CAD build for the part. Positions are in the model's coordinates, mm. A direction names the side the tool comes from. Coordinates: 2 decimals unless noted, no trailing zeros. Order: outer loops, then holes, each group sorted by start corner. A loop starts at its lowest first (then second) coordinate and runs counter-clockwise, first axis right, second up. Notation, with made-up numbers: M 42.25,-20 L 95.25,-20 A21 cw 95.25,3 Z; hole C -3.75,7 d6. An arc over 180 degrees is marked long. Write item = value, one per line. Start each with the question number.
```python
from build123d import *

# Parameters (mm, degrees)
SKETCH_R        = 17.5
PAD_DEPTH       = 58
FILLET_R        = 15
SKETCH001_R     = 14.25
POCKET_DEPTH    = 32
SKETCH002_R     = 1
POCKET001_DEPTH = 58.001
FILLET001_R     = 2


with BuildPart() as part:
    # Sketch → Pad (new body)
    with BuildSketch(Plane.XY):
        Circle(SKETCH_R)
    extrude(amount=PAD_DEPTH)

    # Fillet
    fillet_edges = [part.edges().sort_by_distance(p)[0] for p in [
        (-17.5, 0, 58),
    ]]
    fillet(fillet_edges, radius=FILLET_R)

    # Sketch001 (on Face3 of Fillet) → Pocket (cut)
    with BuildSketch(Plane(origin=(0, 0, 0), x_dir=(1, 0, 0), z_dir=(0, 0, -1))):
        Circle(SKETCH001_R)
    extrude(amount=-POCKET_DEPTH, mode=Mode.SUBTRACT)

    # Sketch002 (on Face4 of Fillet) → Pocket001 (cut, through all)
    with BuildSketch(Plane.XY.offset(58)):
        Circle(SKETCH002_R)
    extrude(amount=-POCKET001_DEPTH, mode=Mode.SUBTRACT)

    # Fillet001
    fillet001_edges = [part.edges().sort_by_distance(p)[0] for p in [
        (-14.25, 0, 0),
    ]]
    fillet(fillet001_edges, radius=FILLET001_R)


solid = part.part
```
1. Slice it at A-A (z = 11). Write the cut outline in (x, y), plus the area to 3 significant figures.
2. Mould opens along Y. For faces 1 (the cylindrical face through (0, -1, 45)), 2 (the cylindrical face through (-13.887, -10.648, 21.199)), 3 (the flat face through (1, -1, 58)) say: released by +Y, released by -Y, zero draft, split by the parting line, or undercut.
3. 3-axis set-ups, long thin cutter, end or side, ignore diameter. For faces 4 (the flat face through (0, 3, 32)), 5 (the flat face through (12, -12, 0)): which of +Z, -Z, +X, -X, +Y, -Y reach the whole face in a straight line?
4. Flat gauge pins, fed straight in: pin 1 (5 mm diameter, centred on x = 11, y = 11, fed in from +Z); pin 2 (3 mm diameter, centred on y = -10.5, z = 28.5, fed in from -X); pin 3 (12 mm diameter, centred on x = 8, y = -6.5, fed in from +Z). Where does each tip first touch, or does it go through?
5. Probe L1, parallel to Y at x = 0, z = 24.5; L2, parallel to Y at x = 0, z = 37; L3, parallel to X at y = -5, z = 29.5. List the from-to ranges inside material, lowest first.
Calculated:
q1.outline = C 0,0 d35; hole C 0,0 d28.5
q1.area = 324 mm²
q2.face_1 = undercut
q2.face_2 = split by the parting line
q2.face_3 = zero draft
q3.face_4 = -Z
q3.face_5 = -Z, +X, -X, +Y, -Y
q4.pin_1 = 53.66
q4.pin_2 = -15.01
q4.pin_3 = 57.89
q5.L1 = -17.5 to -14.25, 14.25 to 17.5
q5.L2 = -17.5 to -1, 1 to 17.5
q5.L3 = -16.77 to -13.34, 13.34 to 16.77
